Build history of the part. All positions in model axes, mm. A direction names the side the tool comes from. Round coordinates to 2 decimals unless told otherwise and drop trailing zeros. Write each loop counter-clockwise with the first axis right and the second up, starting at its lowest first coordinate (ties: lowest second). Pieces come first, ordered by that corner, then holes. Notation, with made-up numbers: M 28,83 L 80,83 A16 cw 80,111 Z; hole C 89,88 d9. An arc over 180 degrees is marked long. Use a Markdown table: item, result.
from build123d import *

# Parameters (mm, degrees)
SKETCH1_R                       = 4.525
SKETCH1_R_2                     = 3.525
BOSS_EXTRUDE1_DEPTH             = 2
SKETCH1_5_R                     = 24.525
SKETCH1_5_R_2                   = 4.525
BOSS_EXTRUDE3_DEPTH             = 3
SKETCH2_R                       = 1.75
CUT_EXTRUDE1_DEPTH              = 4.5
CIRPATTERN1_COUNT               = 3
SKETCH9_W                       = 60
SKETCH9_H                       = 11
BOSS_EXTRUDE7_DEPTH             = 15
BOSS_EXTRUDE7_DIRECTION_2_REACH = 36.813
CUT_EXTRUDE3_REACH              = 54.605
SKETCH10_R                      = 2.5
FILLET4_R                       = 3
FILLET5_R                       = 5


with BuildPart() as part:
    # Sketch1 → Boss-Extrude1 (new body)
    with BuildSketch(Plane(origin=(0, 0, 0), x_dir=(1, 0, 0), z_dir=(0, 1, 0))):
        with Locations(Location((0, 0, 0), (0, 0, 270))):
            Circle(SKETCH1_R)
        with Locations(Location((0, 0, 0), (0, 0, 270))):
            Circle(SKETCH1_R_2, mode=Mode.SUBTRACT)
    extrude(amount=BOSS_EXTRUDE1_DEPTH)

    # Sketch1<5> → Boss-Extrude3 (add)
    with BuildSketch(Plane(origin=(0, 0, 0), x_dir=(1, 0, 0), z_dir=(0, 1, 0))):
        with Locations(Location((0, 0, 0), (0, 0, 270))):
            Circle(SKETCH1_5_R)
        with Locations(Location((0, 0, 0), (0, 0, 270))):
            Circle(SKETCH1_5_R_2, mode=Mode.SUBTRACT)
    extrude(amount=BOSS_EXTRUDE3_DEPTH)

    # Sketch2 → Cut-Extrude1 (cut)
    with BuildSketch(Plane(origin=(0, 3, 0), x_dir=(1, 0, 0), z_dir=(0, 1, 0))):
        with Locations(Location((0, -14.525, 0), (0, 0, 270))):
            Circle(SKETCH2_R)
    cut_extrude1 = extrude(amount=-CUT_EXTRUDE1_DEPTH, mode=Mode.SUBTRACT)

    # CirPattern1: Cut-Extrude1 ×3 about axis
    cirpattern1_axis = Axis((0, 0, 0), (0, 1, 0))
    for i in range(1, CIRPATTERN1_COUNT):
        add(cut_extrude1.rotate(cirpattern1_axis, i * 360 / CIRPATTERN1_COUNT), mode=Mode.SUBTRACT)

    # Sketch9 → Boss-Extrude7 (add)
    with BuildSketch(Plane.XZ):
        with Locations((0, -21.5)):
            Rectangle(SKETCH9_W, SKETCH9_H)
    extrude(amount=BOSS_EXTRUDE7_DEPTH)

    # Boss-Extrude7 direction 2: up to this face of the body (flat: up to its plane)
    boss_extrude7_direction_2_end = Plane(part.part.faces().sort_by_distance((0, 3, -23.831328248))[0])
    # Sketch9 → Boss-Extrude7 direction 2 (add, up to the picked face)
    with BuildSketch(Plane.XZ, mode=Mode.PRIVATE) as boss_extrude7_direction_2_sk1:
        with Locations((0, -21.5)):
            Rectangle(SKETCH9_W, SKETCH9_H)
    boss_extrude7_direction_2_tool1 = split(extrude(boss_extrude7_direction_2_sk1.sketch, amount=-BOSS_EXTRUDE7_DIRECTION_2_REACH, mode=Mode.PRIVATE), bisect_by=boss_extrude7_direction_2_end, keep=Keep.BOTH, mode=Mode.PRIVATE)
    add(boss_extrude7_direction_2_tool1.solids().sort_by(Axis((0, 0, -21.5), (0, 1, 0)))[0])

    # Sketch10 → Cut-Extrude3 (cut, up to next)
    with BuildSketch(Plane.XY.offset(-16), mode=Mode.PRIVATE) as cut_extrude3_sk1:
        with Locations((-18, -7.5)):
            Circle(SKETCH10_R)
    cut_extrude3_tool1 = extrude(cut_extrude3_sk1.sketch, amount=-CUT_EXTRUDE3_REACH, mode=Mode.PRIVATE) & part.part
    # Sketch10 → Cut-Extrude3 (cut, up to next)
    with BuildSketch(Plane.XY.offset(-16), mode=Mode.PRIVATE) as cut_extrude3_sk2:
        with Locations(Location((18, -7.5, 0), (0, 0, 180))):
            Circle(SKETCH10_R)
    cut_extrude3_tool2 = extrude(cut_extrude3_sk2.sketch, amount=-CUT_EXTRUDE3_REACH, mode=Mode.PRIVATE) & part.part
    add(cut_extrude3_tool1.solids().sort_by_distance((-18, -7.5, -16))[0], mode=Mode.SUBTRACT)
    add(cut_extrude3_tool2.solids().sort_by_distance((18, -7.5, -16))[0], mode=Mode.SUBTRACT)

    # Fillet4
    fillet4_edges = [part.edges().sort_by_distance(p)[0] for p in [
        (-30, -6, -16),
        (30, -6, -16),
    ]]
    fillet(fillet4_edges, radius=FILLET4_R)

    # Fillet5
    # the kernel refuses this fillet: 5 mm, written as the material it adds along each edge
    with BuildSketch(Plane(origin=(-18.586974606, 3, -16), x_dir=(-0.999999908254526, 0, -0.0004283584240869523), z_dir=(0, -1, 0))) as fillet5_piece_1:
        with BuildLine():
            CenterArc((8.806331501, -4.993993224), FILLET5_R, 92.808774222, 109.061067494)
            Line((4.166169243, -6.856489993), (3.702153017, -7.04273967))
            ThreePointArc((3.702153017, -7.04273967), (1.938057952, -3.516366711), (-0.379079034, -0.326035406))
            Line((-0.379079034, -0.326035406), (0.000214179, 0.499999954))
            ThreePointArc((0.000214179, 0.499999954), (8.413238801, 0.496396164), (8.536816511, 0.499399322))
            Line((8.536816511, 0.499399322), (8.561317874, 0))
        make_face()
    extrude(amount=3)
    with BuildSketch(Plane(origin=(18.586974606, 3, -16), x_dir=(0.999999908254526, 0, -0.0004283584240865375), z_dir=(0, -1, 0))) as fillet5_piece_2:
        with BuildLine():
            CenterArc((8.806331501, 4.993993224), FILLET5_R, 158.130158283, 109.061067494)
            Line((4.166169243, 6.856489993), (3.702153017, 7.04273967))
            ThreePointArc((3.702153017, 7.04273967), (1.938057952, 3.516366711), (-0.379079034, 0.326035406))
            Line((-0.379079034, 0.326035406), (0.000214179, -0.499999954))
            ThreePointArc((0.000214179, -0.499999954), (8.413238801, -0.496396164), (8.536816511, -0.499399322))
            Line((8.536816511, -0.499399322), (8.561317874, 0))
        make_face()
    extrude(amount=3)


solid = part.part
Q1. Cut at D-D on x = 12.5. Give the cut face in (y, z), and give its area (3 significant figures).
Response values:
| item | result |
|---|---|
| outline | M -15,-27 L 3,-27 L 3,-9.01 L 0,-9.01 L 0,-16 L -15,-16 Z; M 0,-5.51 L 3,-5.51 L 3,21.1 L 0,21.1 Z |
| area | 299 mm2 |
Q2. Cut at B-B on z = 0. Give the cut face in (x, y) (3 decimals).
Response values:
| item | result |
|---|---|
| outline | M -24.525,0 L -3.525,0 L -3.525,2 L -4.525,2 L -4.525,3 L -24.525,3 Z; M 3.525,0 L 24.525,0 L 24.525,3 L 4.525,3 L 4.525,2 L 3.525,2 Z |
Q3. Cut at C-C on y = -7.5. Give the cut face in (x, z).
Response values:
| item | result |
|---|---|
| outline | M -30,-27 L -20.5,-27 L -20.5,-16 L -27,-16 A3 ccw -30,-19 Z; M -15.5,-27 L 15.5,-27 L 15.5,-16 L -15.5,-16 Z; M 20.5,-27 L 30,-27 L 30,-19 A3 ccw 27,-16 L 20.5,-16 Z |
Q4. Which spindle directions (+Z, -Z, +X, -X, +Y, -Y) get a long thin tool onto all of the face, cutting with end or side? Do faces 1 (the cylindrical face through (-20.5, -7.4, -21.4)), 2 (the cylindrical face through (1.359, 2.493, 4.316)), 3 (the flat face through (0, -8, -16)). Say none if no direction does.
Response values:
| item | result |
|---|---|
| face 1 | +Z, -Z |
| face 2 | +Y |
| face 3 | +Z, +X, -X, -Y |
Q5. Drop flat-ended pins along their axis: P1, Ø6.5, axis at x = 0, z = 0, coming from the +Y side; P2, Ø12, axis at x = -15, z = 15.5, coming from the -Y side; P3, Ø1, axis at x = 10, y = -5.5, coming from the +Z side; P4, Ø4.5, axis at x = -1, z = -2, coming from the +Y side. Give the stop position or say it passes through.
Response values:
| item | result |
|---|---|
| P1 | passes through |
| P2 | stops at y = 0 |
| P3 | stops at z = -16 |
| P4 | stops at y = 2 |
Q6. Cut at A-A on x = 0. Give the cut face in (y, z) (3 decimals), and give its area (3 significant figures).
Response values:
| item | result |
|---|---|
| outline | M -15,-27 L 3,-27 L 3,-4.525 L 2,-4.525 L 2,-3.525 L 0,-3.525 L 0,-16 L -15,-16 Z; M 0,3.525 L 2,3.525 L 2,4.525 L 3,4.525 L 3,12.775 L 0,12.775 Z; M 0,16.275 L 3,16.275 L 3,24.525 L 0,24.525 Z |
| area | 286 mm2 |
Q7. Two-plate mould, pull along X, no slides. Class faces 4 (the flat face through (0, -15, -21)), 5 (the cylindrical face through (-29.14, -5.87, -16.9)), 6 (the cylindrical face through (0.077, 1.521, 12.777)): +X half, -X half, draft (parallel to the pull), parting line (faces both ways), or undercut.
Response values:
| item | result |
|---|---|
| face 4 | draft |
| face 5 | -X half |
| face 6 | undercut |
Q8. Drill centre lines: L1, parallel to Y at x = 18, z = -19.25; L2, parallel to X at y = 0.6, z = 0 (3 decimals); L3, parallel to X at y = 2.7, z = 0 (3 decimals). Where is each one in solid material? Low to high.
Response values:
| item | result |
|---|---|
| L1 | y = -15 to -10, -5 to 3 |
| L2 | x = -24.525 to -3.525, 3.525 to 24.525 |
| L3 | x = -24.525 to -4.525, 4.525 to 24.525 |
